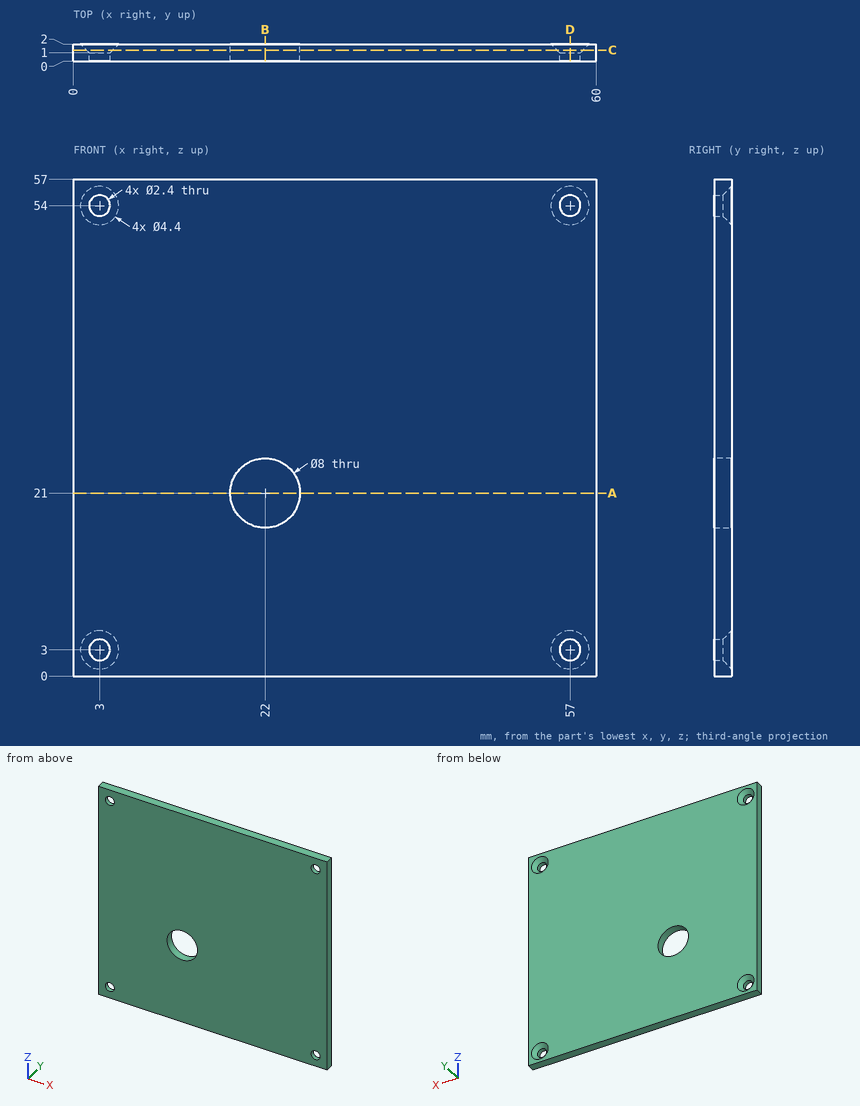
The figure shows three views and two pictorial views of one solid part (mm, origin at its lowest corner). Answer the questions. Give positions to 0.01 mm unless a question says otherwise; leave off trailing zeros. Order: outer loops, then holes, each group sorted by start corner. A loop starts at its lowest first (then second) coordinate and runs counter-clockwise, first axis right, second up. Notation, with made-up numbers: (36.5, -28) - (82.5, -28) arc R24 cw to (82.5, -1) - close; hole circle Ø7 at (-21, -18.5). An arc over 180 degrees is marked (long way). Answer as CSV lines item,"result".
Q1. Straight lines are drawn through the part: L1, parallel to Z at x = 3, y = 0.6; L2, parallel to X at y = 0.65, z = 3; L3, parallel to Z at x = 56, y = 0.6. For each, find the intervals that lie inside material, in ascending order.
Answer key:
L1,"z = 0 to 1.8, 4.2 to 52.8, 55.2 to 57"
L2,"x = 0 to 1.8, 4.2 to 55.8, 58.2 to 60"
L3,"z = 0 to 2.34, 3.66 to 53.34, 54.66 to 57"
Q2. A cutting plane is placed at C-C, the plane y = 1.3. Determine the outline of the cut face in (x, z).
Answer key:
outline,"(0, 0) - (60, 0) - (60, 57) - (0, 57) - close; hole circle Ø3 at (3, 3); hole circle Ø3 at (3, 54); hole circle Ø8 at (22, 21); hole circle Ø3 at (57, 3); hole circle Ø3 at (57, 54)"
Q3. A cutting plane is placed at A-A, the plane z = 21. Determine the outline of the cut face in (x, y).
Answer key:
outline,"(0, 0) - (18, 0) - (18, 2) - (0, 2) - close; (26, 0) - (60, 0) - (60, 2) - (26, 2) - close"
Q4. A cutting plane is placed at D-D, the plane x = 57. Determine the outline of the cut face in (y, z), and give its area (3 significant figures).
Answer key:
outline,"(0, 0) - (2, 0) - (2, 0.8) - (1, 1.8) - (0, 1.8) - close; (0, 4.2) - (1, 4.2) - (2, 5.2) - (2, 51.8) - (1, 52.8) - (0, 52.8) - close; (0, 55.2) - (1, 55.2) - (2, 56.2) - (2, 57) - (0, 57) - close"
area,"102 mm^2"
Q5. Each of these flat-tipped pins is pushed along its axis until it touches: pin 1 Ø3 at (x, z) = (57, 3) entering from +Y; pin 2 Ø8 at (x, z) = (38, 50.5) entering from -Y. Where does it stop, or does it pass through?
Answer key:
pin 1,"stops at y = 1.3"
pin 2,"stops at y = 0"
Q6. A cutting plane is placed at B-B, the plane x = 22. Determine the outline of the cut face in (y, z).
Answer key:
outline,"(0, 0) - (2, 0) - (2, 17) - (0, 17) - close; (0, 25) - (2, 25) - (2, 57) - (0, 57) - close"
